Can you work these out from the model? Positions are in its coordinate system, mm. A direction names the side the tool comes from. Round coordinates to 2 decimals unless told otherwise and drop trailing zeros. Loops run counter-clockwise (first coordinate to the right, second up) from the corner with the lowest first, then second, coordinate; pieces in that order, holes last.
(1) I want a section at B-B on y = 0. Write out the boundary of the cut face in (x, z) (3 decimals).
(2) I want a section at D-D on x = 4.5. Write out the boundary of the cut face in (y, z) (3 decimals), plus the area to 3 significant figures.
(3) Which directions (+Z, -Z, +X, -X, +Y, -Y) give clear straight access to the entire face, cutting with the end or side of a thin tool? Please do faces 1 (the face through (2, -1, 10)), 2 (the face through (-0.37, 2.85, 1.98)), 3 (the face through (-2.5, 0, 10)).
(4) Thinking about a two-plate mould opening in Y: for faces 4 (the face through (0, -2.5, 10)), 5 (the face through (2.5, 0, 10)), 6 (the face through (2, 1, 10)), 7 (the face through (0, 0, 3.5)), which applies, released by +Y, released by -Y, zero draft, split by the parting line, or undercut?
(5) If I drill on line 1 along Y through (x, z) = (0, 2.05) (3 decimals); line 2 along Z through (x, y) = (-0.75, 1.25); line 3 along Y through (x, z) = (-2, 3), over which ranges is the centre line in solid material (lowest first)?
(6) I want a section at A-A on z = 10.25. Write out the boundary of the cut face in (x, y), plus the area to 3 significant figures.
(7) Will these pins go through, and if not, where does the flat tip stop? pin 1 Ø0.8 at (x, z) = (2, 12.5) entering from -Y; pin 2 Ø0.8 at (y, z) = (-1.5, 8.5) entering from -X; pin 3 Ø0.6 at (x, z) = (0.5, 12.5) entering from +Y.
from build123d import *

# Parameters (mm, degrees)
SKETCH1_R           = 4.875
SKETCH1_R_2         = 2.875
BOSS_EXTRUDE1_DEPTH = 3.5
SKETCH2_R           = 4.875
BOSS_EXTRUDE2_DEPTH = 2
CHAMFER1_SIZE       = 0.5
BOSS_EXTRUDE3_DEPTH = 10


with BuildPart() as part:
    # Sketch1 → Boss-Extrude1 (new body)
    with BuildSketch(Plane.XY):
        Circle(SKETCH1_R)
        Circle(SKETCH1_R_2, mode=Mode.SUBTRACT)
    extrude(amount=BOSS_EXTRUDE1_DEPTH)

    # Sketch2 → Boss-Extrude2 (add)
    with BuildSketch(Plane.XY.offset(3.5)):
        Circle(SKETCH2_R)
    extrude(amount=BOSS_EXTRUDE2_DEPTH)

    # Chamfer1
    chamfer1_edges = [part.edges().sort_by_distance(p)[0] for p in [
        (-2.875, 0, 0),
    ]]
    chamfer(chamfer1_edges, length=CHAMFER1_SIZE)

    # Sketch3 → Boss-Extrude3 (add)
    with BuildSketch(Plane.XY.offset(5.5)):
        Polygon((-1, 2.5), (1, 2.5), (1, 1), (2.5, 1), (2.5, -1), (1, -1), (1, -2.5), (-1, -2.5), (-1, -1), (-2.5, -1), (-2.5, 1), (-1, 1), align=None)
    extrude(amount=BOSS_EXTRUDE3_DEPTH)


solid = part.part
Filled sheet:
1. outline: (-4.875, 0) - (-3.375, 0) - (-2.875, 0.5) - (-2.875, 3.5) - (2.875, 3.5) - (2.875, 0.5) - (3.375, 0) - (4.875, 0) - (4.875, 5.5) - (2.5, 5.5) - (2.5, 15.5) - (-2.5, 15.5) - (-2.5, 5.5) - (-4.875, 5.5) - close
2. outline: (-1.875, 0) - (1.875, 0) - (1.875, 5.5) - (-1.875, 5.5) - close
2. area: 20.6 mm2
3. face 1: +Z, +X, -Y
3. face 2: -Z
3. face 3: +Z, -X, +Y, -Y
4. face 4: released by -Y
4. face 5: zero draft
4. face 6: released by +Y
4. face 7: undercut
5. line 1: y = -4.875 to -2.875, 2.875 to 4.875
5. line 2: z = 3.5 to 15.5
5. line 3: y = -4.45 to -2.07, 2.07 to 4.45
6. outline: (-2.5, -1) - (-1, -1) - (-1, -2.5) - (1, -2.5) - (1, -1) - (2.5, -1) - (2.5, 1) - (1, 1) - (1, 2.5) - (-1, 2.5) - (-1, 1) - (-2.5, 1) - close
6. area: 16.0 mm2
7. pin 1: stops at y = -1
7. pin 2: stops at x = -1
7. pin 3: stops at y = 2.5
